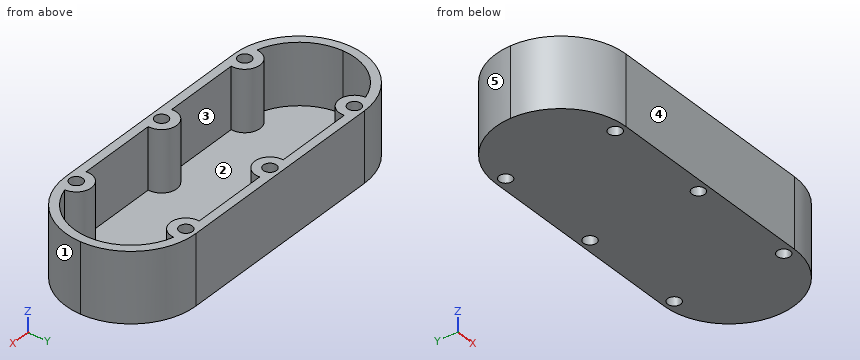
```python
from build123d import *

# Parameters (mm, degrees)
SKETCH3_R           = 1.5
BOSS_EXTRUDE2_DEPTH = 16
SHELL4_T            = -2


with BuildPart() as part:
    # Sketch3 → Boss-Extrude2 (new body)
    with BuildSketch(Plane.XY):
        with BuildLine():
            Line((40.605667182, -0.784898421), (40.605667182, -0.764898421))
            ThreePointArc((40.605667182, -0.764898421), (36.215197832, 9.834632229), (25.615667182, 14.225101579))
            Line((25.615667182, 14.225101579), (-24.404332818, 14.225101579))
            ThreePointArc((-24.404332818, 14.225101579), (-35.003863468, 9.834632229), (-39.394332818, -0.764898421))
            Line((-39.394332818, -0.764898421), (-39.394332818, -0.784898421))
            ThreePointArc((-39.394332818, -0.784898421), (-35.003863468, -11.384429071), (-24.404332818, -15.774898421))
            Line((-24.404332818, -15.774898421), (25.615667182, -15.774898421))
            ThreePointArc((25.615667182, -15.774898421), (36.215197832, -11.384429071), (40.605667182, -0.784898421))
        make_face()
        with Locations(Location((25.569857848, 11.840225967, 0), (0, 0, 180))):
            Circle(SKETCH3_R, mode=Mode.SUBTRACT)
        with Locations(Location((25.615667182, -13.354907477, 0), (0, 0, 180))):
            Circle(SKETCH3_R, mode=Mode.SUBTRACT)
        with Locations(Location((0.19338318, -13.400716811, 0), (0, 0, 180))):
            Circle(SKETCH3_R, mode=Mode.SUBTRACT)
        with Locations(Location((0.605667182, 11.8860353, 0), (0, 0, 180))):
            Circle(SKETCH3_R, mode=Mode.SUBTRACT)
        with Locations(Location((-24.541760819, 11.840225967, 0), (0, 0, 180))):
            Circle(SKETCH3_R, mode=Mode.SUBTRACT)
        with Locations(Location((-24.468118501, -13.332659391, 0), (0, 0, 180))):
            Circle(SKETCH3_R, mode=Mode.SUBTRACT)
    extrude(amount=BOSS_EXTRUDE2_DEPTH)

    # Shell4
    shell4_openings = [part.faces().sort_by_distance(p)[0] for p in [
        (0.60782007, -0.775315064, 16),
    ]]
    offset(amount=SHELL4_T, openings=shell4_openings)


solid = part.part
```
Verification items for the finished model (mm, model axes). Face numbers are marked on the shaded views. A direction names the side the tool comes from. Round coordinates to 2 decimals unless told otherwise and drop trailing zeros. Write each loop counter-clockwise with the first axis right and the second up, starting at its lowest first coordinate (ties: lowest second). Pieces come first, ordered by that corner, then holes.
1. Access from +Z, -Z, +X, -X, +Y, -Y to the whole of each face (thin tool, end or side, straight path). Record for the marked faces 1 and 2.
2. Section check B-B on z = 5.25. State how many separate pieces and enclosed holes the cut face has, plus the area to 3 significant figures.
3. Gauge pin test, flat ends, axial feed: P1, Ø13, axis at x = 11, y = 0, coming from the +Z side; P2, Ø2.5, axis at x = -24.47, y = -13.33, coming from the +Z side; P3, Ø2, axis at x = 32, z = 6, coming from the -Y side. Record the tip position at first contact, or that the pin passes through.
4. Section check C-C on y = 2. Enter the section's corners in (x, z).
5. Scan lines: L1, parallel to Y at x = 19, z = 4.75; L2, parallel to Y at x = -24, z = 1.75; L3, parallel to Y at x = 0.5, z = 10.75. Record each from-to range of solid material in increasing order.
6. Section check A-A on x = -13.5. Enter the section's corners in (y, z), plus the area to 3 significant figures.
7. Draft check along Y on the marked faces 3, 4 and 5. Enter one of: +Y half, -Y half, draft (parallel to the pull), parting line (faces both ways), or undercut.
Answer:
1. face 1: +Z, -Z, +X, -Y
1. face 2: +Z
2. separate pieces: 1
2. enclosed holes: 7
2. area: 463 mm2
3. P1: stops at z = 2
3. P2: passes through
3. P3: stops at y = -14.77
4. outline: (-39.14, 0) - (40.35, 0) - (40.35, 16) - (38.31, 16) - (38.31, 2) - (-37.1, 2) - (-37.1, 16) - (-39.14, 16) - close
5. L1: y = -15.77 to -13.77, 12.23 to 14.23
5. L2: y = -15.77 to -14.76, -11.91 to 10.44, 13.24 to 14.23
5. L3: y = -15.77 to -14.87, -11.93 to -9.91, 8.39 to 10.39, 13.38 to 14.23
6. outline: (-15.77, 0) - (14.23, 0) - (14.23, 16) - (12.23, 16) - (12.23, 2) - (-13.77, 2) - (-13.77, 16) - (-15.77, 16) - close
6. area: 116 mm2
7. face 3: undercut
7. face 4: -Y half
7. face 5: +Y half
